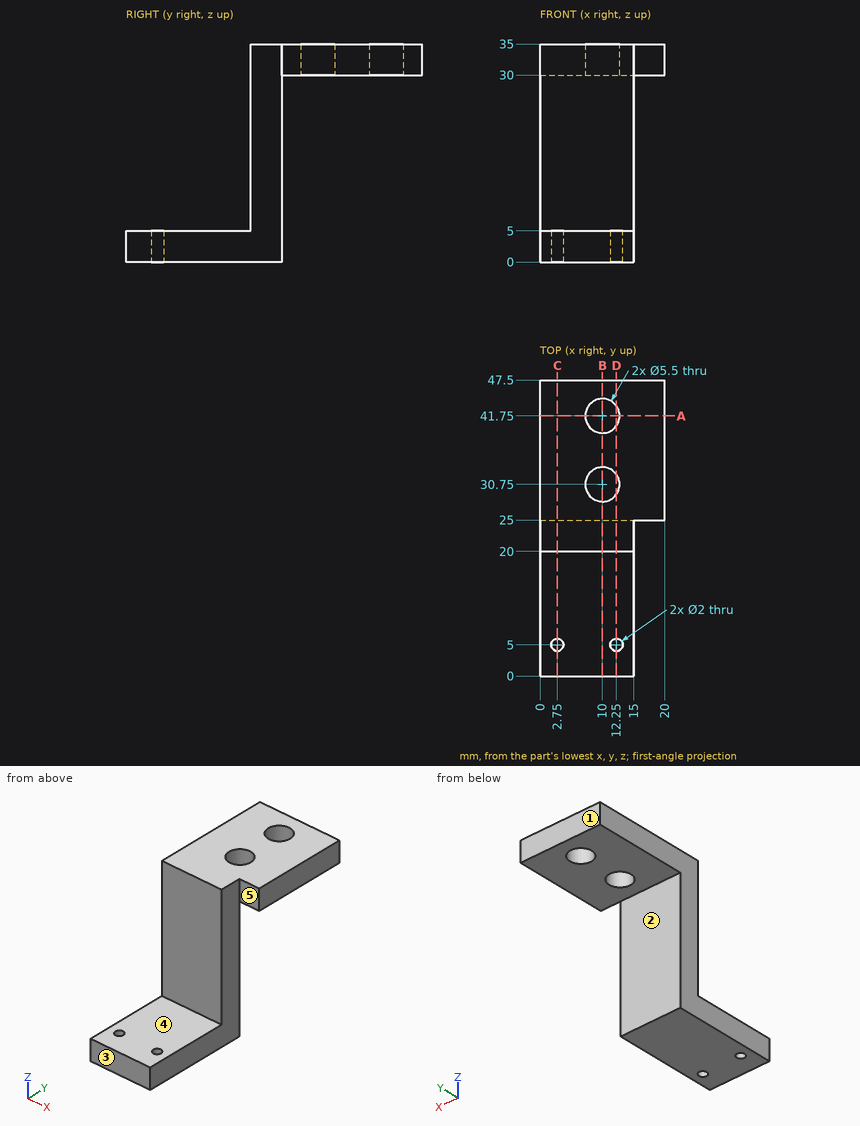
Geometry check sheet. Reference: drawing and pictorial views, mm from the part's lowest x, y, z. A direction names the side the tool comes from. Round coordinates to 2 decimals unless told otherwise and drop trailing zeros. Loops run counter-clockwise (first coordinate to the right, second up) from the corner with the lowest first, then second, coordinate; pieces in that order, holes last. Notation, with made-up numbers: (28, 19) - (65, 19) arc R28 ccw to (65, 43) - close; hole circle Ø2 at (11.5, 75). An arc over 180 degrees is marked (long way). One line per question, with ' | ' between items. Start each with the question number.
1. Cross-section at D-D on x = 12.25. Record the cut outline in (y, z), then the cut area to 3 significant figures.
2. Depth check by flat-ended pin: pin 1 (20 mm diameter, centred on y = 11.5, z = 21, fed in from +X); pin 2 (7.5 mm diameter, centred on x = 7, z = 15, fed in from -Y); pin 3 (4.5 mm diameter, centred on x = 6.5, y = 5.5, fed in from +Z); pin 4 (5 mm diameter, centred on x = 10, y = 41.75, fed in from +Z). Enter the tip coordinate at first touch or a pass-through.
3. Cross-section at A-A on y = 41.75. Record the cut outline in (x, z).
4. Scan lines: line 1 (X direction, y = 5, z = 3.15); line 2 (Y direction, x = 11.75, z = 32.5); line 3 (Z direction, x = 9.5, y = 27). Record each from-to range of solid material in increasing order. Write a range as [from, to].
5. Tool access check on the marked faces 1, 2, 3, 4 and 5. Record the directions out of +Z, -Z, +X, -X, +Y, -Y that give a thin tool (end or side, any length) a straight path to the whole face; none if there is none.
6. Cross-section at B-B on x = 10. Record the cut outline in (y, z), then the cut area to 4 significant figures.
7. Cross-section at C-C on x = 2.75. Record the cut outline in (y, z).
Taken from the geometry:
1) outline: (0, 0) - (4, 0) - (4, 5) - (0, 5) - close; (6, 0) - (25, 0) - (25, 30) - (29.17, 30) - (29.17, 35) - (20, 35) - (20, 5) - (6, 5) - close; (32.33, 30) - (40.17, 30) - (40.17, 35) - (32.33, 35) - close; (43.33, 30) - (47.5, 30) - (47.5, 35) - (43.33, 35) - close | area: 346 mm²
2) pin 1: x = 15 | pin 2: y = 20 | pin 3: z = 5 | pin 4: through
3) outline: (0, 30) - (7.25, 30) - (7.25, 35) - (0, 35) - close; (12.75, 30) - (20, 30) - (20, 35) - (12.75, 35) - close
4) line 1: [0, 1.75], [3.75, 11.25], [13.25, 15] | line 2: [20, 28.63], [32.87, 39.63], [43.87, 47.5] | line 3: [30, 35]
5) face 1: +Z, -Z, +X, -X, +Y | face 2: -Z, +X, -X, +Y | face 3: +Z, -Z, +X, -X, -Y | face 4: +Z, +X, -X, -Y | face 5: +Z, -Z, +X, -Y
6) outline: (0, 0) - (25, 0) - (25, 30) - (28, 30) - (28, 35) - (20, 35) - (20, 5) - (0, 5) - close; (33.5, 30) - (39, 30) - (39, 35) - (33.5, 35) - close; (44.5, 30) - (47.5, 30) - (47.5, 35) - (44.5, 35) - close | area: 332.5 mm²
7) outline: (0, 0) - (4, 0) - (4, 5) - (0, 5) - close; (6, 0) - (25, 0) - (25, 30) - (47.5, 30) - (47.5, 35) - (20, 35) - (20, 5) - (6, 5) - close
